Model file for the job. Use its own axes, mm. Round coordinates to 2 decimals unless told otherwise and drop trailing zeros. Order: outer loops, then holes, each group sorted by start corner. A loop starts at its lowest first (then second) coordinate and runs counter-clockwise, first axis right, second up. Notation, with made-up numbers: (76.25, 16) - (83.25, 16) arc R12 ccw to (83.25, 35) - close; hole circle Ø8 at (58, 35). An arc over 180 degrees is marked (long way). Use one line per item in the form item = value.
from build123d import *

# Parameters (mm, degrees)
SKETCH_1_W             = 12
SKETCH_1_H             = 40
EXTRUDE_1_DEPTH        = 100
HOLE_WIZARD_M6_1_D     = 5
HOLE_WIZARD_M6_1_DEPTH = 15
HOLE_WIZARD_M6_1_TIP   = 1.502151548
HOLE_WIZARD_M8_1_D     = 6.8
CHAMFER_1_SIZE         = 2


with BuildPart() as part:
    # 草图1 → 凸台-拉伸1 (new body)
    with BuildSketch(Plane(origin=(0, 0, 0), x_dir=(1, 0, 0), z_dir=(0, 1, 0))):
        Rectangle(SKETCH_1_W, SKETCH_1_H)
    extrude(amount=EXTRUDE_1_DEPTH)

    # M6 螺纹孔1
    with Locations(Plane(origin=(0, 100, 0), x_dir=(1, 0, 0), z_dir=(0, 1, 0))):
        with Locations((0, 15), (0, -15)):
            Hole(HOLE_WIZARD_M6_1_D / 2, depth=HOLE_WIZARD_M6_1_DEPTH)
            with Locations((0, 0, -(HOLE_WIZARD_M6_1_DEPTH + HOLE_WIZARD_M6_1_TIP / 2))):  # 118° drill point
                Cone(0, HOLE_WIZARD_M6_1_D / 2, HOLE_WIZARD_M6_1_TIP, mode=Mode.SUBTRACT)

    # M8 螺纹孔1 (through all)
    with Locations(Plane(origin=(6, 0, 0), x_dir=(0, 0, -1), z_dir=(1, 0, 0))):
        with Locations((0, 15)):
            Hole(HOLE_WIZARD_M8_1_D / 2)

    # 倒角1
    chamfer_1_edges = [part.edges().sort_by_distance(p)[0] for p in [
        (0, 0, 20),
        (0, 0, -20),
    ]]
    chamfer(chamfer_1_edges, length=CHAMFER_1_SIZE)


solid = part.part
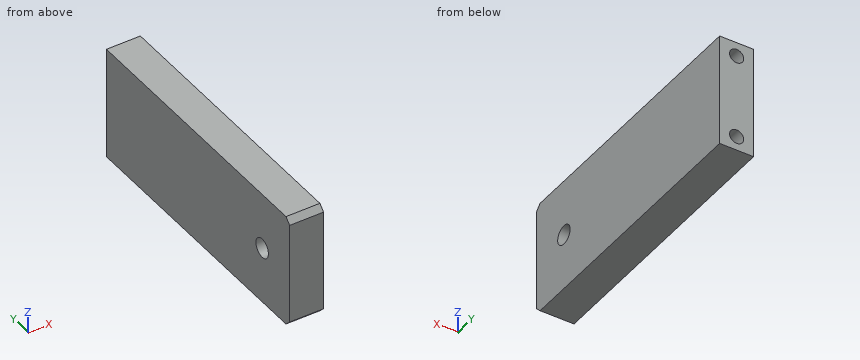
(1) Probe probe 1 along Z at (x, y) = (0, 92.75); probe 2 along X at (y, z) = (96.5, -15); probe 3 along Y at (x, z) = (5.5, 3). List the from-to ranges inside material, lowest first. Write a range as [from, to].
Report:
probe_1 = [-20, -17.5], [-12.5, 12.5], [17.5, 20]
probe_2 = [-6, -2.5], [2.5, 6]
probe_3 = [0, 13.4], [16.6, 100]
(2) Pin check, flat tip, straight feed: pin 1 (4 mm diameter, centred on x = 0, z = -15, fed in from +Y). Stop position of the tip, or through.
Report:
pin_1 = 84.7
(3) Slice it at A-A on z = 0. Give the cut face in (x, y), then the cut area to 3 significant figures.
Report:
outline = (-6, 0) - (6, 0) - (6, 11.6) - (-6, 11.6) - close; (-6, 18.4) - (6, 18.4) - (6, 100) - (-6, 100) - close
area = 1,120 mm2
